from build123d import *
from OCP.BRepFilletAPI import BRepFilletAPI_MakeChamfer

# Parameters (mm, degrees)
SKETCH1_R           = 5.75
BOSS_EXTRUDE1_DEPTH = 3
BOSS_EXTRUDE2_DEPTH = 0.15
CIRPATTERN1_COUNT   = 2
SKETCH4_R           = 2.5
CUT_EXTRUDE1_DEPTH  = 65.150588849
CHAMFER2_SIZE       = 1
CHAMFER2_SIZE2      = 1.191753593


with BuildPart() as part:
    # Sketch1 → Boss-Extrude1 (new, symmetric)
    with BuildSketch(Plane(origin=(0, 0, 0), x_dir=(1, 0, 0), z_dir=(0, 1, 0))):
        with Locations(Location((0, 0, 0), (0, 0, 270))):
            Circle(SKETCH1_R)
    extrude(amount=BOSS_EXTRUDE1_DEPTH, both=True)

    # Sketch3 → Boss-Extrude2 (add, symmetric)
    with BuildSketch(Plane(origin=(0, 0, 0), x_dir=(0.9743700647852351, -0.2249510543438655, 0), z_dir=(-0.2249510543438655, -0.9743700647852351, 0))):
        with BuildLine():
            Line((-4.594330289, 1.95406384), (-7.004950747, 5.194012526))
            Line((-7.004950747, 5.194012526), (-7.004950747, 60.5))
            ThreePointArc((-7.004950747, 60.5), (-6.12627109, 62.621320344), (-4.004950747, 63.5))
            Line((-4.004950747, 63.5), (-3.349097477, 63.5))
            ThreePointArc((-3.349097477, 63.5), (-0.196862037, 62.381161132), (1.54463599, 59.525364693))
            add(Edge.make_bspline(
                [(1.54463599, 59.525364693), (9.475219296, 30.694015203), (4.834288523, 1.046023407)],
                knots=[0, 0, 0, 1, 1, 1], degree=2))
            add(Edge.make_bspline(
                [(-4.594330289, 1.95406384), (0.469577579, 8.859977358), (4.834288523, 1.046023407)],
                knots=[0, 0, 0, 1, 1, 1], degree=2))
        make_face()
    boss_extrude2 = extrude(amount=BOSS_EXTRUDE2_DEPTH, both=True)

    # CirPattern1: Boss-Extrude2 ×2 about axis
    cirpattern1_axis = Axis((0, 3, 0), (0, -1, 0))
    for i in range(1, CIRPATTERN1_COUNT):
        add(boss_extrude2.rotate(cirpattern1_axis, i * 360 / CIRPATTERN1_COUNT))

    # Sketch4 → Cut-Extrude1 (cut, through all)
    with BuildSketch(Plane.XZ.offset(3)):
        with Locations(Location((0, 0, 0), (0, 0, 270))):
            Circle(SKETCH4_R)
    extrude(amount=-CUT_EXTRUDE1_DEPTH, mode=Mode.SUBTRACT)

    # Chamfer2: one chamfer whose edges measure the first distance from different faces: ONE call of the kernel's chamfer builder (chamfer() names one face for all edges)
    chamfer2_edges_1 = [part.edges().sort_by_distance(p)[0] for p in [
        (0, 3, 2.5),
    ]]
    chamfer2_side_1 = [part.faces().sort_by_distance(p)[0] for p in [
        (0, 0, 2.5),
    ]]
    chamfer2_edges_2 = [part.edges().sort_by_distance(p)[0] for p in [
        (0, -3, 2.5),
    ]]
    chamfer2_side_2 = [part.faces().sort_by_distance(p)[0] for p in [
        (0, -3, -5.58736544),
    ]]
    chamfer2 = BRepFilletAPI_MakeChamfer(part.part.solid().wrapped)
    for e in chamfer2_edges_1:
        chamfer2.Add(CHAMFER2_SIZE, CHAMFER2_SIZE2, e.wrapped, chamfer2_side_1[0].wrapped)  # the first distance lies on this face
    for e in chamfer2_edges_2:
        chamfer2.Add(CHAMFER2_SIZE, CHAMFER2_SIZE2, e.wrapped, chamfer2_side_2[0].wrapped)  # the first distance lies on this face
    add(Compound.cast(chamfer2.Shape()), mode=Mode.REPLACE)


solid = part.part
Input: part model. Units: mm. Frame: model coordinates. A direction names the side the tool comes from. Coordinates: 2 decimals unless noted, no trailing zeros. Order: outer loops, then holes, each group sorted by start corner. A loop starts at its lowest first (then second) coordinate and runs counter-clockwise, first axis right, second up. Notation, with made-up numbers: M 77,-11 L 100,-11 A36 cw 100,28 Z; hole C 39,-7.75 d5. An arc over 180 degrees is marked long. One line per question, with ' | ' between items.
Item 1: Pin query (flat end, axial travel): pin 1 (5 mm diameter, centred on x = 0.5, z = 16.5, fed in from +Y); pin 2 (1.5 mm diameter, centred on x = -5, z = 14, fed in from +Y); pin 3 (3 mm diameter, centred on x = 4.5, z = -29, fed in from -Y). Return the tip coordinate at first contact, or that it passes through.
Geometry results:
pin 1: stops at y = 0.62 | pin 2: stops at y = 1.48 | pin 3: stops at y = 0.54
Item 2: Reachability of faces 1 (the flat face through (0, -3, 4)), 2 (the cylindrical face through (1.727, 0.042, 5.484)) from +Z, -Z, +X, -X, +Y, -Y: full face, straight path, thin tool, end or side. Return the list, or none.
Geometry results:
face 1: +Z, -Z, +X, -X, -Y | face 2: none
Item 3: Draft query along X for faces 3 (the cylindrical face through (-2.44, 0.07, 0.54)), 4 (the flat face through (-4, 3, 0)). Return one class per face: released by +X, released by -X, zero draft, split by the parting line, or undercut.
Geometry results:
face 3: undercut | face 4: zero draft
Item 4: Ray query, line 1 along X through (y, z) = (0.65, 0); line 2 along Y through (x, z) = (-3, 25); line 3 along Y through (x, z) = (-5, -7). Return the intervals inside material, ascending.
Geometry results:
line 1: x = -5.75 to -2.5, 2.5 to 5.75 | line 2: y = 0.54 to 0.85 | line 3: y = -1.31 to -1
Item 5: Section A-A (z = 0). Output: boundary loops of the cut face in (x, y).
Geometry results:
outline: M -5.75,-3 L -3.5,-3 L -2.5,-1.81 L -2.5,2 L -3.69,3 L -5.75,3 Z; M 2.5,-1.81 L 3.5,-3 L 5.75,-3 L 5.75,3 L 3.69,3 L 2.5,2 Z
